For this review, use the dimensioned drawing (mm, ordinates from the lowest corner) and the shaded views. A direction names the side the tool comes from. Coordinates: 2 decimals unless noted, no trailing zeros. Loops run counter-clockwise (first coordinate to the right, second up) from the corner with the lowest first, then second, coordinate; pieces in that order, holes last. Notation, with made-up numbers: (73, 39) - (131, 39) arc R9 ccw to (131, 47) - close; hole circle Ø11 at (-5, 56.5). An arc over 180 degrees is marked (long way). Answer in a Markdown table with one row per item. Add a question column.
(1) We need section B-B on x = 19. Write out the cut boundary in (y, z).
(2) We need section C-C on y = 36. Write out the cut boundary in (x, z).
(3) Mouldability with a two-part tool opening along X and no side actions: class the marked faces 3, 4 and 5 as +X half, -X half, draft (parallel to the pull), parting line (faces both ways), or undercut.
(4) We need section D-D on x = 9. Write out the cut boundary in (y, z), plus the area to 3 significant figures.
(5) We need section A-A on z = 31. Write out the cut boundary in (x, y).
(6) Machinability: for the marked faces 1 and 2, which of the approach directions +Z, -Z, +X, -X, +Y, -Y give a long, thin tool a straight path to every point of the face, cutting with its end or side? Answer none if there is none.
(7) For P1, Ø10, axis at x = 20.5, y = 23, coming from the +Z side; P2, Ø1.5, axis at x = 13, z = 34.5, coming from the -Y side; P3, Ø7.5, axis at x = 22.68, z = 32.93, coming from the -Y side, all flat-tipped, find the tip position at first contact; note any pin that passes through.
(8) For line 1 along Z through (x, y) = (7.5, 19); line 2 along Y through (x, z) = (41, 31), list the stretches that pass through material, from the lowest coordinate up.
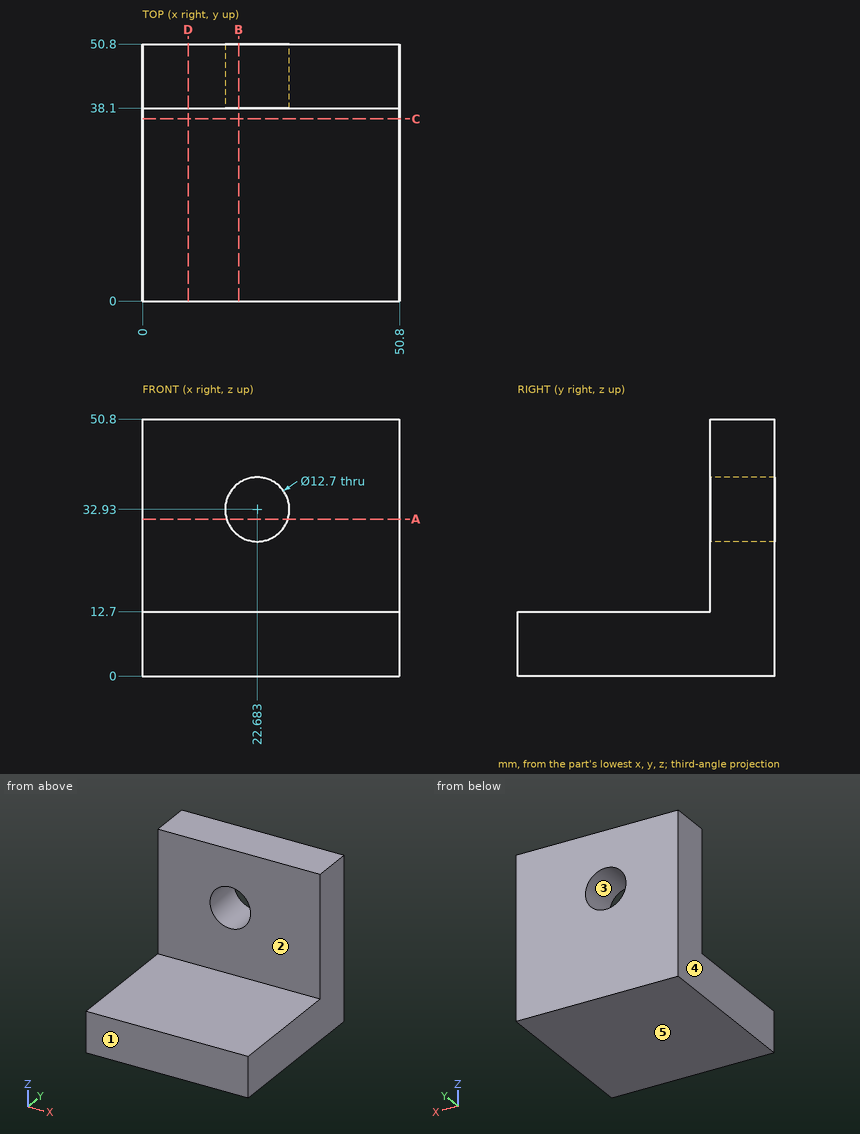
Outcome:
| question | item | result |
|---|---|---|
| 1 | outline | (0, 0) - (50.8, 0) - (50.8, 27.76) - (38.1, 27.76) - (38.1, 12.7) - (0, 12.7) - close; (38.1, 38.1) - (50.8, 38.1) - (50.8, 50.8) - (38.1, 50.8) - close |
| 2 | outline | (0, 0) - (50.8, 0) - (50.8, 12.7) - (0, 12.7) - close |
| 3 | face 3 | undercut |
| 3 | face 4 | -X half |
| 3 | face 5 | draft |
| 4 | outline | (0, 0) - (50.8, 0) - (50.8, 50.8) - (38.1, 50.8) - (38.1, 12.7) - (0, 12.7) - close |
| 4 | area | 1,130 mm² |
| 5 | outline | (0, 38.1) - (16.63, 38.1) - (16.63, 50.8) - (0, 50.8) - close; (28.73, 38.1) - (50.8, 38.1) - (50.8, 50.8) - (28.73, 50.8) - close |
| 6 | face 1 | +Z, -Z, +X, -X, -Y |
| 6 | face 2 | +Z, +X, -X, -Y |
| 7 | P1 | z = 12.7 |
| 7 | P2 | y = 38.1 |
| 7 | P3 | through |
| 8 | line 1 | 0 to 12.7 |
| 8 | line 2 | 38.1 to 50.8 |
